Check sheet for the modelled part. Datum: model origin and axes. Units: mm. Give positions to 0.01 mm unless a question says otherwise; leave off trailing zeros. Loops run counter-clockwise (first coordinate to the right, second up) from the corner with the lowest first, then second, coordinate; pieces in that order, holes last. Notation, with made-up numbers: (19.25, -20) - (50.25, -20) arc R20 cw to (50.25, -7) - close; hole circle Ø4 at (-3, 65.5). An arc over 180 degrees is marked (long way). Answer in a Markdown table with one row per item. Add a question column.
(1) Draft check along Z on faces 1 (the face through (51.2, 1.5, -20.8)), 2 (the face through (115, 1, -32)), 3 (the face through (0.86, 1.52, -64.1)). Enter one of: released by +Z, released by -Z, zero draft, split by the parting line, or undercut.
(2) Sectioned sample at C-C on y = 1.7. State how many separate pieces and enclosed holes the cut face has, then the cut area to 3 significant figures.
(3) Sectioned sample at A-A on z = -5. Enter the section's corners in (x, y), then the cut area to 3 significant figures.
(4) Go/stop test with a flat-tipped pin: P1, Ø7, axis at x = 5, z = -60, coming from the -Y side. Record where the tip stops, or that it passes through.
(5) Sectioned sample at B-B on x = 110. Enter the section's corners in (y, z), then the cut area to 3 significant figures.
(6) Sectioned sample at D-D on z = -22.5. Enter the section's corners in (x, y), then the cut area to 3 significant figures.
(7) Thickness scan on L1, parallel to X at y = 0.9, z = -45; L2, parallel to X at y = 1.4, z = -20; L3, parallel to X at y = 1.5, z = -60. Record the ranges inside material, lowest first.
from build123d import *

# Parameters (mm, degrees)
SKETCH1_W            = 115
SKETCH1_H            = 65
BOSS_EXTRUDE1_DEPTH  = 3
SKETCH2_R            = 6.25
CUT_EXTRUDE1_DEPTH   = 3
LPATTERN1_COUNT      = 4
LPATTERN1_PITCH      = 25
LPATTERN1_COUNT_DIR2 = 2
LPATTERN1_PITCH_DIR2 = 25
SKETCH3_R            = 8.25
CUT_EXTRUDE2_DEPTH   = 3
M5_CLEARANCE_HOLE1_D = 5.3
FILLET1_R            = 3


with BuildPart() as part:
    # Sketch1 → Boss-Extrude1 (new body)
    with BuildSketch(Plane(origin=(0, 0, 0), x_dir=(1, 0, 0), z_dir=(0, 1, 0))):
        with Locations((57.5, 32.5)):
            Rectangle(SKETCH1_W, SKETCH1_H)
    extrude(amount=BOSS_EXTRUDE1_DEPTH)

    # Sketch2 → Cut-Extrude1 (cut)
    with BuildSketch(Plane(origin=(0, 3, 0), x_dir=(1, 0, 0), z_dir=(0, 1, 0))):
        with Locations(Location((20, 20, 0), (0, 0, 270))):
            Circle(SKETCH2_R)
    cut_extrude1 = extrude(amount=-CUT_EXTRUDE1_DEPTH, mode=Mode.SUBTRACT)

    # LPattern1: Cut-Extrude1 4 × 2, 2 skipped
    with Locations(*[(i * LPATTERN1_PITCH, 0, -j * LPATTERN1_PITCH_DIR2) for i in range(LPATTERN1_COUNT) for j in range(LPATTERN1_COUNT_DIR2) if (i, j) not in ((0, 0), (1, 1), (2, 1))]):
        add(cut_extrude1, mode=Mode.SUBTRACT)

    # Sketch3 → Cut-Extrude2 (cut)
    with BuildSketch(Plane(origin=(0, 3, 0), x_dir=(1, 0, 0), z_dir=(0, 1, 0))):
        with Locations(Location((45, 45, 0), (0, 0, 270))):
            Circle(SKETCH3_R)
        with Locations(Location((70, 45, 0), (0, 0, 270))):
            Circle(SKETCH3_R)
    extrude(amount=-CUT_EXTRUDE2_DEPTH, mode=Mode.SUBTRACT)

    # M5 Clearance Hole1 (through all)
    with Locations(Plane(origin=(0, 3, 0), x_dir=(1, 0, 0), z_dir=(0, 1, 0))):
        with Locations((5, 60), (5, 5), (110, 5), (110, 60)):
            Hole(M5_CLEARANCE_HOLE1_D / 2)

    # Fillet1
    fillet1_edges = [part.edges().sort_by_distance(p)[0] for p in [
        (0, 1.5, -65),
        (115, 1.5, -65),
        (115, 1.5, 0),
        (0, 1.5, 0),
    ]]
    fillet(fillet1_edges, radius=FILLET1_R)


solid = part.part
Reply:
| question | item | result |
|---|---|---|
| 1 | face 1 | undercut |
| 1 | face 2 | zero draft |
| 1 | face 3 | released by -Z |
| 2 | separate pieces | 1 |
| 2 | enclosed holes | 12 |
| 2 | area | 6,220 mm^2 |
| 3 | outline | (0, 0) - (2.35, 0) - (2.35, 3) - (0, 3) - close; (7.65, 0) - (107.35, 0) - (107.35, 3) - (7.65, 3) - close; (112.65, 0) - (115, 0) - (115, 3) - (112.65, 3) - close |
| 3 | area | 313 mm^2 |
| 4 | P1 | y = 0 |
| 5 | outline | (0, -65) - (3, -65) - (3, -62.65) - (0, -62.65) - close; (0, -57.35) - (3, -57.35) - (3, -7.65) - (0, -7.65) - close; (0, -2.35) - (3, -2.35) - (3, 0) - (0, 0) - close |
| 5 | area | 163 mm^2 |
| 6 | outline | (0, 0) - (14.27, 0) - (14.27, 3) - (0, 3) - close; (25.73, 0) - (39.27, 0) - (39.27, 3) - (25.73, 3) - close; (50.73, 0) - (64.27, 0) - (64.27, 3) - (50.73, 3) - close; (75.73, 0) - (89.27, 0) - (89.27, 3) - (75.73, 3) - close; (100.73, 0) - (115, 0) - (115, 3) - (100.73, 3) - close |
| 6 | area | 208 mm^2 |
| 7 | L1 | 0 to 13.75, 26.25 to 36.75, 53.25 to 61.75, 78.25 to 88.75, 101.25 to 115 |
| 7 | L2 | 0 to 13.75, 26.25 to 38.75, 51.25 to 63.75, 76.25 to 88.75, 101.25 to 115 |
| 7 | L3 | 0 to 2.35, 7.65 to 107.35, 112.65 to 115 |
